Here's the drawing with two shaded views (mm, measured from the low corner). I have some questions. A direction names the side the tool comes from. Coordinates: 2 decimals unless noted, no trailing zeros. Loops run counter-clockwise (first coordinate to the right, second up) from the corner with the lowest first, then second, coordinate; pieces in that order, holes last. Notation, with made-up numbers: (-38, -40) - (-31, -40) arc R25 cw to (-31, -17) - close; hole circle Ø9 at (-19, -28). An arc over 180 degrees is marked (long way). Use a Markdown table: item, result.
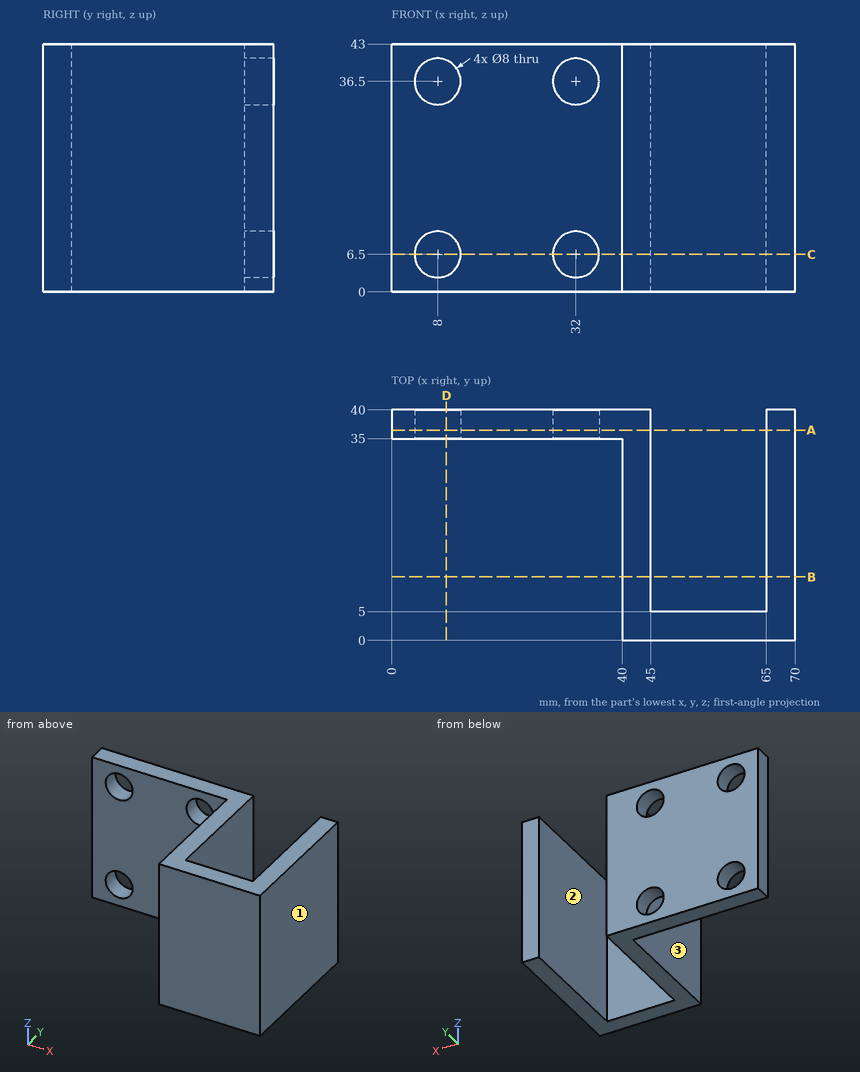
Q1. I want a section at B-B, the plane y = 11. Write out the boundary of the cut face in (x, z), then the cut area to 3 significant figures.
Check values:
| item | result |
|---|---|
| outline | (40, 0) - (45, 0) - (45, 43) - (40, 43) - close; (65, 0) - (70, 0) - (70, 43) - (65, 43) - close |
| area | 430 mm^2 |
Q2. I want a section at D-D, the plane x = 9.5. Write out the boundary of the cut face in (y, z), then the cut area to 3 significant figures.
Check values:
| item | result |
|---|---|
| outline | (35, 0) - (40, 0) - (40, 2.79) - (35, 2.79) - close; (35, 10.21) - (40, 10.21) - (40, 32.79) - (35, 32.79) - close; (35, 40.21) - (40, 40.21) - (40, 43) - (35, 43) - close |
| area | 141 mm^2 |
Q3. I want a section at A-A, the plane y = 36.5. Write out the boundary of the cut face in (x, z), then the cut area to 3 significant figures.
Check values:
| item | result |
|---|---|
| outline | (0, 0) - (45, 0) - (45, 43) - (0, 43) - close; (65, 0) - (70, 0) - (70, 43) - (65, 43) - close; hole circle Ø8 at (8, 6.5); hole circle Ø8 at (8, 36.5); hole circle Ø8 at (32, 6.5); hole circle Ø8 at (32, 36.5) |
| area | 1,950 mm^2 |
Q4. I want a section at C-C, the plane z = 6.5. Write out the boundary of the cut face in (x, y), then the cut area to 3 significant figures.
Check values:
| item | result |
|---|---|
| outline | (0, 35) - (4, 35) - (4, 40) - (0, 40) - close; (12, 35) - (28, 35) - (28, 40) - (12, 40) - close; (36, 35) - (40, 35) - (40, 0) - (70, 0) - (70, 40) - (65, 40) - (65, 5) - (45, 5) - (45, 40) - (36, 40) - close |
| area | 620 mm^2 |
Q5. Which directions (+Z, -Z, +X, -X, +Y, -Y) give clear straight access to the entire face, cutting with the end or side of a thin tool? Please do the marked faces 1, 2 and 3.
Check values:
| item | result |
|---|---|
| face 1 | +Z, -Z, +X, +Y, -Y |
| face 2 | +Z, -Z, +Y |
| face 3 | +Z, -Z, -X, -Y |
Q6. Please list where these lines run through material, in increasing order: L1, parallel to X at y = 38.6, z = 36.5; L2, parallel to X at y = 31.5, z = 40.5; L3, parallel to X at y = 38, z = 19. Write a range as from..to.
Check values:
| item | result |
|---|---|
| L1 | 0..4, 12..28, 36..45, 65..70 |
| L2 | 40..45, 65..70 |
| L3 | 0..45, 65..70 |
Q7. Will these pins go through, and if not, where does the flat tip stop? P1, Ø17.5, axis at y = 23, z = 18, coming from the -X side; P2, Ø6, axis at x = 56.5, z = 20.5, coming from the +Y side; P3, Ø12, axis at x = 20, z = 27, coming from the -Y side.
Check values:
| item | result |
|---|---|
| P1 | x = 40 |
| P2 | y = 5 |
| P3 | y = 35 |
